Solid Edge part; units mm, degrees
sketch "Sketch1" plane through (0, 0, 0) normal (0, -1, 0) x (1, 0, 0)
  line L0 (22.5, 36.5) -> (22.5, -19)
  line L1 (22.5, -19) -> (-22.5, -19)
  line L2 (-22.5, -19) -> (-22.5, 36.5)
  line L3 (-22.5, 36.5) -> (22.5, 36.5)
  circle A0 centre (0, 28) radius 6
  circle A1 centre (0, 8) radius 4.6
extrude "Protrusion1" add sketch "Sketch1" against normal blind 10
sketch "Sketch2" plane through (0, 10, 4.6) normal (0, 1, 0) x (-1, 0, 0)
  circle A0 centre (0, 3.4) radius 11.25
extrude "ExtrudedCutout_1" cut sketch "Sketch2" against normal blind 7.5
sketch "Sketch3" plane through (0, 2.5, 8) normal (0, 1, 0) x (-1, 0, 0)
  circle A0 centre (0, 0) radius 4.6
extrude "Protrusion2" add sketch "Sketch3" against normal up to vertex (2.5 mm away)
sketch "Sketch4" plane through (0, 0, 0) normal (0, -1, 0) x (1, 0, 0)
  circle A0 centre (-16, -14) radius 2.25
  circle A1 centre (16, -14) radius 2.25
extrude "Cutout1" cut sketch "Sketch4" against normal up to next
The listing builds one solid part. Answer for the finished solid, in the listing's coordinates (mm). A direction names the side the tool comes from. Give positions to 0.01 mm unless a question says otherwise; leave off trailing zeros. Loops run counter-clockwise (first coordinate to the right, second up) from the corner with the lowest first, then second, coordinate; pieces in that order, holes last. Notation, with made-up numbers: M 84,30.5 L 105,30.5 A35 cw 105,68.5 Z; hole C -28.75,2.25 d7. An arc over 180 degrees is marked long. One line per item, written item: value.
1. This flat-tipped pin is pushed along its axis until it touches: P1, Ø5, axis at x = -0.5, z = 3.5, coming from the +Y side. Where does it stop, or does it pass through?
Found:
P1: y = 2.5
2. Find the intervals of material crossed by probe 1 along Z at (x, y) = (0, 7.5); probe 2 along Z at (x, y) = (1.5, 3); probe 3 along X at (y, z) = (4.5, 28.5), in increasing order.
Found:
probe 1: -19 to -3.25, 19.25 to 22, 34 to 36.5
probe 2: -19 to -3.15, 19.15 to 22.19, 33.81 to 36.5
probe 3: -22.5 to -5.98, 5.98 to 22.5
3. Section D-D on z = 8 is taken. Determine the outline of the cut face in (x, y).
Found:
outline: M -22.5,0 L 22.5,0 L 22.5,10 L 11.25,10 L 11.25,2.5 L -11.25,2.5 L -11.25,10 L -22.5,10 Z
4. Section A-A on x = 0 is taken. Determine the outline of the cut face in (y, z), plus the area to 3 significant figures.
Found:
outline: M 0,-19 L 10,-19 L 10,-3.25 L 2.5,-3.25 L 2.5,19.25 L 10,19.25 L 10,22 L 0,22 Z; M 0,34 L 10,34 L 10,36.5 L 0,36.5 Z
area: 266 mm^2
5. For faces 1 (the face through (0, 5, -19)), 2 (the face through (0, 2.5, 8)), determine the directions among +Z, -Z, +X, -X, +Y, -Y from which every point of the face is accessible in a straight line to the end or side of a thin tool.
Found:
face 1: -Z, +X, -X, +Y, -Y
face 2: +Y
6. Section B-B on z = 28 is taken. Determine the outline of the cut face in (x, y), plus the area to 3 significant figures.
Found:
outline: M -22.5,0 L -6,0 L -6,10 L -22.5,10 Z; M 6,0 L 22.5,0 L 22.5,10 L 6,10 Z
area: 330 mm^2
7. For a pull along X with two mould halves and no side action, classify faces 3 (the face through (22.5, 5, 9)), 4 (the face through (18.146, 4.93, -13.324)), 5 (the face through (0, 10, -4)) as pulls with the +X half, pulls with the -X half, needs draft (parallel to the pull), parting line crosses it, or undercut.
Found:
face 3: pulls with the +X half
face 4: undercut
face 5: needs draft
8. Section C-C on y = 7.75 is taken. Determine the outline of the cut face in (x, z), plus the area to 3 significant figures.
Found:
outline: M -22.5,-19 L 22.5,-19 L 22.5,36.5 L -22.5,36.5 Z; hole C -16,-14 d4.5; hole C 0,8 d22.5; hole C 0,28 d12; hole C 16,-14 d4.5
area: 1,950 mm^2
